from build123d import *

# Parameters (mm, degrees)
F0_R      = 6.95
F1_DEPTH  = 2.3
F2_R      = 2.575
F3_DEPTH  = 3.6
F4_R      = 6.95
F5_DEPTH  = 2.3
F6_R      = 3.3
F7_DEPTH  = 3.8
F10_R     = 2.5
F11_DEPTH = 3.8


with BuildPart() as f1:
    # F0 (on Top) → F1 (new body)
    with BuildSketch(Plane.XY):
        Circle(F0_R)
    extrude(amount=F1_DEPTH)

    # F2 (on face) → F3 (join)
    with BuildSketch(Plane.XY.offset(2.3)):
        Circle(F2_R)
    extrude(amount=F3_DEPTH)

    # F4 (on face) → F5 (join)
    with BuildSketch(Plane.XY.offset(5.9)):
        Circle(F4_R)
    extrude(amount=F5_DEPTH)

    # F6 (on face) → F7 (join)
    with BuildSketch(Plane.XY.offset(8.2)):
        Circle(F6_R)
    extrude(amount=F7_DEPTH)

    # F8 (on Front) → F9 (revolve)
    with BuildSketch(Plane.XZ):
        with BuildLine():
            ThreePointArc((-3.3, 12), (-3.6249137921, 10.5), (-3.3, 9))
            Line((-3.3, 9), (-3.3, 12))
        make_face()
    revolve(axis=Axis((0, 0, 8.2), (0, 0, -1)))

    # F10 (on face) → F11 (cut, through all)
    with BuildSketch(Plane.XY.offset(12)):
        Circle(F10_R)
    extrude(amount=-F11_DEPTH, mode=Mode.SUBTRACT)


solid = f1.part
The listing builds one solid part. Answer for the finished solid, in the listing's coordinates (mm). A direction names the side the tool comes from. Round coordinates to 2 decimals unless told otherwise and drop trailing zeros. Order: outer loops, then holes, each group sorted by start corner. A loop starts at its lowest first (then second) coordinate and runs counter-clockwise, first axis right, second up. Notation, with made-up numbers: (27.25, -10.5) -> (65.25, -10.5) arc R17 cw to (65.25, 5.5) -> close; hole circle Ø1 at (36, -8). An arc over 180 degrees is marked (long way). Put each result on its own line as item: value.
Q1. Determine the mould class of faces 4 (the flat face through (0, 0, 8.2)), 5 (the flat face through (0, 0, 0)), 6 (the cylindrical face through (2.456, 0.773, 4.075)) for opening direction Y: pulls with the +Y half, pulls with the -Y half, needs draft (parallel to the pull), parting line crosses it, or undercut.
Results list:
face 4: undercut
face 5: needs draft
face 6: parting line crosses it
Q2. Consider line 1 along Z through (x, y) = (-1.75, 3.75); line 2 along Z through (x, y) = (-2, 2.25); line 3 along Z through (x, y) = (-1.5, -3). Determine where each line is inside the solid, lowest interval first.
Results list:
line 1: 0 to 2.3, 5.9 to 8.2
line 2: 0 to 2.3, 5.9 to 12
line 3: 0 to 2.3, 5.9 to 8.2, 9.13 to 11.87
Q3. Section A-A, the plane x = 0 is taken. Write down the section's boundary in (y, z) (3 decimals).
Results list:
outline: (-6.95, 0) -> (6.95, 0) -> (6.95, 2.3) -> (2.575, 2.3) -> (2.575, 5.9) -> (6.95, 5.9) -> (6.95, 8.2) -> (3.3, 8.2) -> (3.3, 9) arc R3.625 ccw to (3.3, 12) -> (2.5, 12) -> (2.5, 8.2) -> (-2.5, 8.2) -> (-2.5, 12) -> (-3.3, 12) arc R3.625 ccw to (-3.3, 9) -> (-3.3, 8.2) -> (-6.95, 8.2) -> (-6.95, 5.9) -> (-2.575, 5.9) -> (-2.575, 2.3) -> (-6.95, 2.3) -> close
Q4. Section C-C, the plane x = -5.5 is taken. Write down the section's boundary in (y, z).
Results list:
outline: (-4.25, 0) -> (4.25, 0) -> (4.25, 2.3) -> (-4.25, 2.3) -> close; (-4.25, 5.9) -> (4.25, 5.9) -> (4.25, 8.2) -> (-4.25, 8.2) -> close
Q5. Each of these flat-tipped pins is pushed along its axis until it touches: P1, Ø1.5, axis at x = 0, y = -1, coming from the +Z side; P2, Ø2, axis at y = -0.5, z = 4.5, coming from the -X side (3 decimals); P3, Ø6, axis at y = 4.5, z = 7.5, coming from the -X side. Where does it stop, or does it pass through?
Results list:
P1: z = 8.2
P2: x = -2.575
P3: x = -6.79
Q6. Which of the six approach directions +Z, -Z, +X, -X, +Y, -Y give full straight-line access (tool end or side, diameter ignored) to faces 1 (the cylindrical face through (-1.507, -6.785, 1.134)), 2 (the cylindrical face through (-0.54, -2.44, 10.13)), 3 (the flat face through (3, 0, 5.9))?
Results list:
face 1: +Z, -Z
face 2: +Z
face 3: none
Q7. Section B-B, the plane y = 5.75 is taken. Write down the section's boundary in (x, z).
Results list:
outline: (-3.9, 0) -> (3.9, 0) -> (3.9, 2.3) -> (-3.9, 2.3) -> close; (-3.9, 5.9) -> (3.9, 5.9) -> (3.9, 8.2) -> (-3.9, 8.2) -> close
Q8. Section D-D, the plane z = 1 is taken. Write down the section's boundary in (x, y), and give its area (3 significant figures).
Results list:
outline: circle Ø13.9 at (0, 0)
area: 152 mm^2
